```python
from build123d import *

# Parameters (mm, degrees)
BOSS_EXTRUDE1_DEPTH   = 5
SKETCH1_W             = 35
SKETCH1_H             = 5
BOSS_EXTRUDE1_2_DEPTH = 5
SKETCH2_W             = 56.57205094
SKETCH2_H             = 46.29963395
CUT_EXTRUDE1_DEPTH    = 10
BOSS_EXTRUDE2_DEPTH   = 5
SKETCH4_W             = 15
SKETCH4_H             = 10
CUT_EXTRUDE2_DEPTH    = 5


with BuildPart() as part:
    # Sketch1 → Boss-Extrude1 (new body)
    with BuildSketch(Plane.XY):
        with BuildLine():
            Line((-45, 70), (0, 70))
            Line((0, 70), (0, 330))
            Line((0, 330), (-5.4, 330))
            Line((-5.4, 330), (-5.4, 323.2))
            Line((-5.4, 323.2), (-4, 323.2))
            Line((-4, 323.2), (-4, 320))
            Line((-4, 320), (-5.4, 320))
            Line((-5.4, 320), (-5.4, 313))
            Line((-5.4, 313), (-9.6, 313))
            Line((-9.6, 313), (-9.6, 320))
            Line((-9.6, 320), (-11, 320))
            Line((-11, 320), (-11, 323.2))
            Line((-11, 323.2), (-9.6, 323.2))
            Line((-9.6, 323.2), (-9.6, 330))
            Line((-9.6, 330), (-20, 330))
            Line((-20, 330), (-20, 335))
            Line((-20, 335), (-55, 335))
            Line((-55, 335), (-55, 330))
            Line((-55, 330), (-65.4, 330))
            Line((-65.4, 330), (-65.4, 323.2))
            Line((-65.4, 323.2), (-64, 323.2))
            Line((-64, 323.2), (-64, 320))
            Line((-64, 320), (-65.4, 320))
            Line((-65.4, 320), (-65.4, 313))
            Line((-65.4, 313), (-69.6, 313))
            Line((-69.6, 313), (-69.6, 320))
            Line((-69.6, 320), (-71, 320))
            Line((-71, 320), (-71, 323.2))
            Line((-71, 323.2), (-69.6, 323.2))
            Line((-69.6, 323.2), (-69.6, 330))
            Line((-69.6, 330), (-80, 330))
            Line((-80, 330), (-80, 335))
            Line((-80, 335), (-90, 335))
            Line((-90, 335), (-90, 330))
            Line((-90, 330), (-92.9, 330))
            Line((-92.9, 330), (-92.9, 323.2))
            Line((-92.9, 323.2), (-91.5, 323.2))
            Line((-91.5, 323.2), (-91.5, 320))
            Line((-91.5, 320), (-92.9, 320))
            Line((-92.9, 320), (-92.9, 313))
            Line((-92.9, 313), (-97.1, 313))
            Line((-97.1, 313), (-97.1, 320))
            Line((-97.1, 320), (-98.5, 320))
            Line((-98.5, 320), (-98.5, 323.2))
            Line((-98.5, 323.2), (-97.1, 323.2))
            Line((-97.1, 323.2), (-97.1, 330))
            Line((-97.1, 330), (-100, 330))
            Line((-100, 330), (-100, 335))
            Line((-100, 335), (-110, 335))
            Line((-110, 335), (-110, -5))
            Line((-110, -5), (-100, -5))
            Line((-100, -5), (-100, 0))
            Line((-100, 0), (-97.1, 0))
            Line((-97.1, 0), (-97.1, 6.8))
            Line((-97.1, 6.8), (-98.5, 6.8))
            Line((-98.5, 6.8), (-98.5, 10))
            Line((-98.5, 10), (-97.1, 10))
            Line((-97.1, 10), (-97.1, 17))
            Line((-97.1, 17), (-92.9, 17))
            Line((-92.9, 17), (-92.9, 10))
            Line((-92.9, 10), (-91.5, 10))
            Line((-91.5, 10), (-91.5, 6.8))
            Line((-91.5, 6.8), (-92.9, 6.8))
            Line((-92.9, 6.8), (-92.9, 0))
            Line((-92.9, 0), (-90, 0))
            Line((-90, 0), (-90, -5))
            Line((-90, -5), (-80, -5))
            Line((-80, -5), (-80, 35))
            ThreePointArc((-80, 35), (-69.748737342, 59.748737342), (-45, 70))
        make_face()
    extrude(amount=BOSS_EXTRUDE1_DEPTH)

    # Sketch3 → Boss-Extrude2 (add)
    with BuildSketch(Plane.XY.offset(5)):
        with BuildLine():
            Line((0, 305), (25, 305))
            Line((25, 305), (25, 70))
            Line((25, 70), (25, -5))
            Line((25, -5), (10, -5))
            Line((10, -5), (10, 35))
            ThreePointArc((10, 35), (-0.251262658, 59.748737342), (-25, 70))
            Line((-25, 70), (0, 70))
            Line((0, 70), (0, 305))
        make_face()
    extrude(amount=-BOSS_EXTRUDE2_DEPTH)

    # Sketch4 → Cut-Extrude2 (cut)
    with BuildSketch(Plane.XY.offset(5)):
        with Locations((17.5, 0)):
            Rectangle(SKETCH4_W, SKETCH4_H)
    extrude(amount=-CUT_EXTRUDE2_DEPTH, mode=Mode.SUBTRACT)


with BuildPart() as body_2:
    # Sketch1 → Boss-Extrude1 2 (new body)
    with BuildSketch(Plane.XY):
        with Locations((-37.5, -2.5)):
            Rectangle(SKETCH1_W, SKETCH1_H)
    extrude(amount=BOSS_EXTRUDE1_2_DEPTH)

    # Sketch2 → Cut-Extrude1 (cut)
    with BuildSketch(Plane.XY.offset(5)):
        with Locations((-32.79534341, -6.148476698)):
            Rectangle(SKETCH2_W, SKETCH2_H)
    extrude(amount=-CUT_EXTRUDE1_DEPTH, mode=Mode.SUBTRACT)


solid = part.part
```
Work out the finished part from the listing and answer in its coordinate system (mm). Coordinates: 2 decimals unless noted, no trailing zeros. Loops run counter-clockwise (first coordinate to the right, second up) from the corner with the lowest first, then second, coordinate; pieces in that order, holes last.
1) Consider probe 1 along Y at (x, z) = (-92, 2.3); probe 2 along X at (y, z) = (20, 4.25); probe 3 along Y at (x, z) = (-40, 0.8). Determine where each line is inside the solid, lowest interval first.
Results:
probe 1: y = 0 to 6.8, 10 to 320, 323.2 to 330
probe 2: x = -110 to -80, 10 to 25
probe 3: y = 70 to 335
2) For a pull along X with two mould halves and no side action, classify faces 1 (the cylindrical face through (-70.019, 59.475, 2.465)), 2 (the cylindrical face through (0.019, 59.475, 2.535)), 3 (the flat face through (-42, 205, 5)) as +X half, -X half, draft (parallel to the pull), parting line (faces both ways), or undercut.
Results:
face 1: undercut
face 2: undercut
face 3: draft
3) Section B-B (x = 14) is taken. Give the vertices of the cut face in (y, z).
Results:
outline: (5, 0) - (305, 0) - (305, 5) - (5, 5) - close
4) Flat-ended cylindrical pins translate along their axes: pin 1 (1 mm diameter, centred on y = 322, z = 1.5, fed in from +X); pin 2 (1.5 mm diameter, centred on x = -35.5, z = 2, fed in from -Y); pin 3 (1.5 mm diameter, centred on y = 332.5, z = 3, fed in from +X). Find the tip coordinate at first contact, or state that the pin passes through.
Results:
pin 1: stops at x = 0
pin 2: stops at y = 70
pin 3: stops at x = -20
5) Section A-A (x = -28) is taken. Give the vertices of the cut face in (y, z), plus the area to 4 significant figures.
Results:
outline: (70, 0) - (335, 0) - (335, 5) - (70, 5) - close
area: 1,325 mm2
